Work out the finished part from the listing and answer in its coordinate system (mm). A direction names the side the tool comes from. Round coordinates to 2 decimals unless told otherwise and drop trailing zeros. Loops run counter-clockwise (first coordinate to the right, second up) from the corner with the lowest first, then second, coordinate; pieces in that order, holes last. Notation, with made-up numbers: M 31,83 L 47,83 A27 ccw 47,109 Z; hole C 21,-2.75 d5. An arc over 180 degrees is marked long. One line per item, written item: value.
```python
from build123d import *

# Parameters (mm, degrees)
F0_W        = 80
F0_H        = 43
F1_DEPTH    = 4
F2_W        = 78
F2_H        = 41
F3_DEPTH    = 12
F4_R        = 5
F5_R        = 0.5
F6_R        = 2
F7_T1_DEPTH = 12
F7_T4_ANGLE = 90
F11_R       = 2.5
F12_DEPTH   = 0.25
F13_DEPTH   = 5
F14_R       = 2.375
F15_DEPTH   = 0.3
F16_R       = 0.25
F17_DEPTH   = 0.5


# Not quite as in the source:
# - a fillet or chamfer that OpenCascade refuses, or shapes differently, is made with other operations: its cross-section is extruded or revolved along the edge and cut away or added


with BuildPart() as f1:
    # F0 (on Top) → F1 (new body)
    with BuildSketch(Plane.XY):
        with Locations((40, 21.5)):
            Rectangle(F0_W, F0_H)
    extrude(amount=F1_DEPTH)

    # F2 (on face) → F3 (join)
    with BuildSketch(Plane.XY.offset(4)):
        with Locations((39, 20.5)):
            Rectangle(F2_W, F2_H)
    extrude(amount=F3_DEPTH)

    # F4
    f4_edges = [f1.edges().sort_by_distance(p)[0] for p in [
        (80, 43, 2),
    ]]
    fillet(f4_edges, radius=F4_R)

    # F5
    f5_edges = [f1.edges().sort_by_distance(p)[0] for p in [
        (37.5, 43, 4),
        (78.535534, 41.535534, 4),
        (80, 19, 4),
    ]]
    fillet(f5_edges, radius=F5_R)

    # F6
    f6_edges = [f1.edges().sort_by_distance(p)[0] for p in [
        (78, 20.5, 16),
        (39, 41, 16),
    ]]
    fillet(f6_edges, radius=F6_R)

    # F7: fillet of radius 4 on 1 edges, made by hand

    # F7_s2 → F7_t1 (cut)
    with BuildSketch(Plane.XY.offset(4)):
        with BuildLine():
            ThreePointArc((74, 41), (76.8284271247, 39.8284271247), (78, 37))
            Line((78, 37), (78, 41))
            Line((78, 41), (74, 41))
        make_face()
    extrude(amount=F7_T1_DEPTH, mode=Mode.SUBTRACT)

    # F7_s3 → F7_t4 (revolve, cut)
    with BuildSketch(Plane.XZ.offset(-37)):
        with BuildLine():
            ThreePointArc((76, 16), (77.4142135624, 15.4142135624), (78, 14))
            Line((78, 14), (78, 16))
            Line((78, 16), (76, 16))
        make_face()
    revolve(axis=Axis((74, 37, 16), (0, 0, 1)), revolution_arc=F7_T4_ANGLE, mode=Mode.SUBTRACT)

    # F8: F1 across face


with BuildPart() as f1_1:
    add(f1.part)
    add(f1.part.mirror(Plane(origin=(39.2268461901, 0, 7.956765433), x_dir=(1, 0, 0), z_dir=(0, -1, 0))))

    # F9: F1 across face


with BuildPart() as f1_2:
    add(f1_1.part)
    add(f1_1.part.mirror(Plane(origin=(0, 0, 7.9181659321), x_dir=(0, -1, 0), z_dir=(-1, 0, 0))))

    # F10: F1 across face


with BuildPart() as f1_3:
    add(f1_2.part)
    add(f1_2.part.mirror(Plane(origin=(0, 0, 0), x_dir=(1, 0, 0), z_dir=(0, 0, -1))))

    # F11 (on face) → F12 (cut)
    with BuildSketch(Plane.YZ.offset(80)):
        with Locations((-34, 0)):
            Circle(F11_R)
    extrude(amount=-F12_DEPTH, mode=Mode.SUBTRACT)

    # F11 (on face) → F13 (cut)
    with BuildSketch(Plane.YZ.offset(80)):
        with BuildLine():
            Line((-24, -1.5), (-16, -1.5))
            ThreePointArc((-16, -1.5), (-14.5, 0), (-16, 1.5))
            Line((-16, 1.5), (-24, 1.5))
            ThreePointArc((-24, 1.5), (-25.5, 0), (-24, -1.5))
        make_face()
        with BuildLine():
            Line((-4, -1.5), (4, -1.5))
            ThreePointArc((4, -1.5), (5.5, 0), (4, 1.5))
            Line((4, 1.5), (-4, 1.5))
            ThreePointArc((-4, 1.5), (-5.5, 0), (-4, -1.5))
        make_face()
        with BuildLine():
            Line((16, -1.5), (24, -1.5))
            ThreePointArc((24, -1.5), (25.5, 0), (24, 1.5))
            Line((24, 1.5), (16, 1.5))
            ThreePointArc((16, 1.5), (14.5, 0), (16, -1.5))
        make_face()
    extrude(amount=-F13_DEPTH, mode=Mode.SUBTRACT)

    # F14 (on face) → F15 (join)
    with BuildSketch(Plane.YZ.offset(79.75)):
        with Locations((-34, 0)):
            Circle(F14_R)
    extrude(amount=F15_DEPTH)

    # F16 (on face) → F17 (cut)
    with BuildSketch(Plane.YZ.offset(80)):
        with Locations((-21.2721988683, 3)):
            Circle(F16_R)
        with Locations((-18.2721988683, 3)):
            Circle(F16_R)
        with Locations((-16.7721988683, 3)):
            Circle(F16_R)
        with Locations((-22.7721988683, 3)):
            Circle(F16_R)
        with Locations((-24.2721988683, 3)):
            Circle(F16_R)
        with Locations((-19.7721988683, 3)):
            Circle(F16_R)
    extrude(amount=-F17_DEPTH, mode=Mode.SUBTRACT)


solid = f1_3.part
```
1) Find section B-B (y = -34). Give the vertices of the cut face in (x, z) (3 decimals).
Check values:
outline: M -80,-3.5 A0.5 ccw -79.5,-4 L -78,-4 L -78,-14 A2 ccw -76,-16 L 76,-16 A2 ccw 78,-14 L 78,-4 L 79.5,-4 A0.5 ccw 80,-3.5 L 80,-2.5 L 79.75,-2.5 L 79.75,-2.375 L 80.05,-2.375 L 80.05,2.375 L 79.75,2.375 L 79.75,2.5 L 80,2.5 L 80,3.5 A0.5 ccw 79.5,4 L 78,4 L 78,14 A2 ccw 76,16 L -76,16 A2 ccw -78,14 L -78,4 L -79.5,4 A0.5 ccw -80,3.5 Z
2) Each of these flat-tipped pins is pushed along its axis until it touches: pin 1 (2 mm diameter, centred on y = -19.5, z = 9.5, fed in from -X); pin 2 (2 mm diameter, centred on x = 47, z = -9.5, fed in from -Y); pin 3 (11 mm diameter, centred on y = -9.5, z = -8.5, fed in from +X). Where does it stop, or does it pass through?
Check values:
pin 1: x = -78
pin 2: y = -41
pin 3: x = 80
3) Find the intervals of material crossed by probe 1 along X at (y, z) = (35, 10); probe 2 along Y at (x, z) = (16.5, 6); probe 3 along X at (y, z) = (-38.5, -10.5), in increasing order. Write a range as from..to.
Check values:
probe 1: -78..78
probe 2: -41..41
probe 3: -77.71..77.71
4) For faces 4 (the face through (78, 20, -1.5)), 5 (the face through (1, -41, 9)), 6 (the face through (78, 1, 9)), determine the directions among +Z, -Z, +X, -X, +Y, -Y from which every point of the face is accessible in a straight line to the end or side of a thin tool.
Check values:
face 4: +X
face 5: +Z, +X, -X, -Y
face 6: +Z, +X, +Y, -Y
5) Find section C-C (z = -10.5). Give the vertices of the cut face in (x, y), then the cut area to 3 significant figures.
Check values:
outline: M -78,-37 A4 ccw -74,-41 L 74,-41 A4 ccw 78,-37 L 78,37 A4 ccw 74,41 L -74,41 A4 ccw -78,37 Z
area: 12,800 mm2
6) The mould has two halves that part along Y. Classify faces 1 (the face through (1, -41, -9)), 2 (the face through (78, 0, 1.5)), 3 (the face through (1, -1, -16)): +Y half, -Y half, draft (parallel to the pull), parting line (faces both ways), or undercut.
Check values:
face 1: -Y half
face 2: undercut
face 3: draft
7) Find section A-A (x = -23). Give the vertices of the cut face in (y, z).
Check values:
outline: M -43,-3.5 A0.5 ccw -42.5,-4 L -41,-4 L -41,-14 A2 ccw -39,-16 L 39,-16 A2 ccw 41,-14 L 41,-4 L 42.5,-4 A0.5 ccw 43,-3.5 L 43,3.5 A0.5 ccw 42.5,4 L 41,4 L 41,14 A2 ccw 39,16 L -39,16 A2 ccw -41,14 L -41,4 L -42.5,4 A0.5 ccw -43,3.5 Z
